from build123d import *

# Parameters (mm, degrees)
SKETCH1_R                = 1.6
BOSS_EXTRUDE1_DEPTH      = 20
BOSS_EXTRUDE2_DEPTH      = 2
SKETCH1_4_W              = 21.213203436
SKETCH1_4_H              = 2
BOSS_EXTRUDE3_DEPTH      = 2
BOSS_EXTRUDE3_DEPTH_BACK = 2


with BuildPart() as part:
    # Sketch1 → Boss-Extrude1 (new body)
    with BuildSketch(Plane(origin=(0, 0, 0), x_dir=(1, 0, 0), z_dir=(0, 1, 0))):
        Polygon((-7.071067812, -14.142135624), (14.142135624, 7.071067812), (7.071067812, 14.142135624), (-14.142135624, -7.071067812), align=None)
        Circle(SKETCH1_R, mode=Mode.SUBTRACT)
    extrude(amount=BOSS_EXTRUDE1_DEPTH)

    # Sketch1_3 → Boss-Extrude2 (add)
    with BuildSketch(Plane(origin=(0, 0, 0), x_dir=(1, 0, 0), z_dir=(0, 1, 0))):
        Polygon((14.142135624, 7.071067812), (-7.071067812, -14.142135624), (-7.071067812, -15.1), (14.142135624, -15.1), align=None)
    extrude(amount=BOSS_EXTRUDE2_DEPTH)

    # Sketch1_4 → Boss-Extrude3 (add, two sides)
    with BuildSketch(Plane(origin=(0, 0, 0), x_dir=(1, 0, 0), z_dir=(0, 1, 0))) as boss_extrude3_sk:
        with Locations((3.535533906, -16.1)):
            Rectangle(SKETCH1_4_W, SKETCH1_4_H)
    extrude(amount=BOSS_EXTRUDE3_DEPTH)
    extrude(boss_extrude3_sk.sketch, amount=-BOSS_EXTRUDE3_DEPTH_BACK)


solid = part.part
The model under review builds one solid part; all positions refer to its coordinate system, in mm. A direction names the side the tool comes from. Give positions to 0.01 mm unless a question says otherwise; leave off trailing zeros. Write each loop counter-clockwise with the first axis right and the second up, starting at its lowest first coordinate (ties: lowest second). Pieces come first, ordered by that corner, then holes.
1. Draft analysis for pull direction X (two halves, no side actions). For faces 1 (the flat face through (6, 2, 8)), 2 (the flat face through (-3.39, 9.86, -3.68)), 3 (the cylindrical face through (-1.27, 9.86, 0.97)), state which applies: +X half, -X half, draft (parallel to the pull), parting line (faces both ways), or undercut.
2. Wall thickness on L1, parallel to Z at x = 0, y = 10; L2, parallel to Y at x = 12, z = -2: over which ranges is each line inside the solid? List them lowest first.
3. Add section B-B, the plane z = 0. Write out the cut boundary in (x, y), plus the area to 3 significant figures.
4. Add section D-D, the plane x = 11. Write out the cut boundary in (y, z), plus the area to 3 significant figures.
5. For P1, Ø6, axis at y = 17, z = -1, coming from the -X side; P2, Ø4, axis at x = 7, y = 12, coming from the +Z side; P3, Ø2, axis at x = -0.5, y = 2, coming from the -Z side; P4, Ø1, axis at x = -5.5, z = 13, coming from the +Y side, all flat-tipped, find the tip position at first contact; note any pin that passes through.
6. Add section C-C, the plane y = 9. Write out the cut boundary in (x, z), plus the area to 3 significant figures.
7. Add section A-A, the plane x = 0. Write out the cut boundary in (y, z), plus the area to 3 significant figures.
8. Tool access review of faces 4 (the flat face through (10.656, 9.86, -10.557)), 5 (the flat face through (3.39, 10.87, 3.68)), 6 (the flat face through (3, 0, 4)), 7 (the flat face through (-7.071, 0, 16)): name each direction out of +Z, -Z, +X, -X, +Y, -Y from which nothing blocks a thin tool from reaching the whole face with its end or side.
Worked answers:
1. face 1: draft
1. face 2: -X half
1. face 3: undercut
2. L1: z = -7.07 to -1.6, 1.6 to 7.07
2. L2: y = 0 to 2
3. outline: (-7.07, 0) - (-1.6, 0) - (-1.6, 20) - (-7.07, 20) - close; (1.6, 0) - (14.14, 0) - (14.14, 2) - (7.07, 2) - (7.07, 20) - (1.6, 20) - close
3. area: 233 mm2
4. outline: (-2, 15.1) - (0, 15.1) - (0, -10.21) - (20, -10.21) - (20, -3.93) - (2, -3.93) - (2, 17.1) - (-2, 17.1) - close
4. area: 172 mm2
5. P1: stops at x = -9.07
5. P2: stops at z = 2.07
5. P3: stops at z = -7.57
5. P4: stops at y = 20
6. outline: (-14.14, 7.07) - (7.07, -14.14) - (14.14, -7.07) - (-7.07, 14.14) - close; hole circle Ø3.2 at (0, 0)
6. area: 292 mm2
7. outline: (-2, 15.1) - (0, 15.1) - (0, 1.6) - (20, 1.6) - (20, 7.07) - (2, 7.07) - (2, 17.1) - (-2, 17.1) - close; (0, -7.07) - (20, -7.07) - (20, -1.6) - (0, -1.6) - close
7. area: 243 mm2
8. face 4: -Z, +X, +Y, -Y
8. face 5: +Z, +X, +Y
8. face 6: -Z, +X, -X, -Y
8. face 7: +Z, -X, +Y, -Y
